Geometry check sheet. Reference: the model listing, model coordinates, mm. Face numbers are marked on the shaded views. A direction names the side the tool comes from. Round coordinates to 2 decimals unless told otherwise and drop trailing zeros. Order: outer loops, then holes, each group sorted by start corner. A loop starts at its lowest first (then second) coordinate and runs counter-clockwise, first axis right, second up.
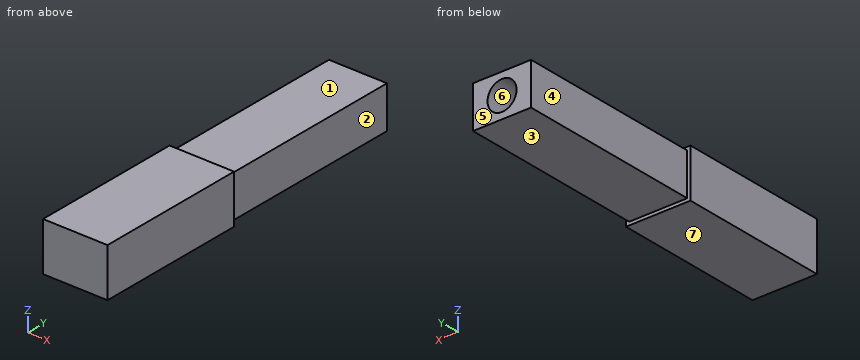
```python
from build123d import *

# Parameters (mm, degrees)
SKETCH1_W           = 20
SKETCH1_H           = 15
BOSS_EXTRUDE1_DEPTH = 47
SKETCH2_W           = 18
SKETCH2_H           = 13
BOSS_EXTRUDE2_DEPTH = 58
SKETCH3_R           = 4.5
CUT_EXTRUDE1_DEPTH  = 58


with BuildPart() as part:
    # Sketch1 → Boss-Extrude1 (new body)
    with BuildSketch(Plane(origin=(0, 0, 0), x_dir=(1, 0, 0), z_dir=(0, 1, 0))):
        with Locations((10, 7.5)):
            Rectangle(SKETCH1_W, SKETCH1_H)
    extrude(amount=BOSS_EXTRUDE1_DEPTH)

    # Sketch2 → Boss-Extrude2 (add)
    with BuildSketch(Plane(origin=(0, 47, 0), x_dir=(1, 0, 0), z_dir=(0, 1, 0))):
        with Locations((10, 7.5)):
            Rectangle(SKETCH2_W, SKETCH2_H)
    extrude(amount=BOSS_EXTRUDE2_DEPTH)

    # Sketch3 → Cut-Extrude1 (cut)
    with BuildSketch(Plane(origin=(0, 105, 0), x_dir=(1, 0, 0), z_dir=(0, 1, 0))):
        with Locations((10, 7.5)):
            Circle(SKETCH3_R)
    extrude(amount=-CUT_EXTRUDE1_DEPTH, mode=Mode.SUBTRACT)


solid = part.part
```
(1) Sectioned sample at C-C, the plane z = -7.5. Record the cut outline in (x, y), and give its area (3 significant figures).
Returned:
outline: (0, 0) - (20, 0) - (20, 47) - (19, 47) - (19, 105) - (14.5, 105) - (14.5, 47) - (5.5, 47) - (5.5, 105) - (1, 105) - (1, 47) - (0, 47) - close
area: 1,460 mm2
(2) Sectioned sample at A-A, the plane x = 10. Record the cut outline in (y, z).
Returned:
outline: (0, -15) - (47, -15) - (47, -14) - (105, -14) - (105, -12) - (47, -12) - (47, -3) - (105, -3) - (105, -1) - (47, -1) - (47, 0) - (0, 0) - close
(3) Draft check along Z on the marked faces 5, 6 and 7. Enter one of: released by +Z, released by -Z, zero draft, split by the parting line, or undercut.
Returned:
face 5: zero draft
face 6: undercut
face 7: released by -Z
(4) Sectioned sample at D-D, the plane x = 4.25. Record the cut outline in (y, z).
Returned:
outline: (0, -15) - (47, -15) - (47, -14) - (105, -14) - (105, -1) - (47, -1) - (47, 0) - (0, 0) - close
(5) Depth check by flat-ended pin: P1, Ø8, axis at x = 11.5, y = 78.5, coming from the +Z side; P2, Ø5, axis at y = 83.5, z = -5, coming from the -X side; P3, Ø7, axis at x = 10, z = -7.5, coming from the +Y side. Enter the tip coordinate at first touch or a pass-through.
Returned:
P1: stops at z = -1
P2: stops at x = 1
P3: stops at y = 47
(6) Material ranges on line 1 (Z direction, x = 10, y = 71); line 2 (X direction, y = 88.5, z = -7.5); line 3 (Z direction, x = 3.75, y = 59.5), recorded low to high.
Returned:
line 1: z = -14 to -12, -3 to -1
line 2: x = 1 to 5.5, 14.5 to 19
line 3: z = -14 to -1
(7) Set-up check for the marked faces 1, 2, 3 and 4: record each of +Z, -Z, +X, -X, +Y, -Y from which the full face is reachable in a straight line by a thin tool's end or side.
Returned:
face 1: +Z, +X, -X, +Y
face 2: +Z, -Z, +X, +Y
face 3: -Z, +X, -X, +Y
face 4: +Z, -Z, -X, +Y
(8) Sectioned sample at B-B, the plane y = 76.5. Record the cut outline in (x, z), and give its area (3 significant figures).
Returned:
outline: (1, -14) - (19, -14) - (19, -1) - (1, -1) - close; hole circle Ø9 at (10, -7.5)
area: 170 mm2
